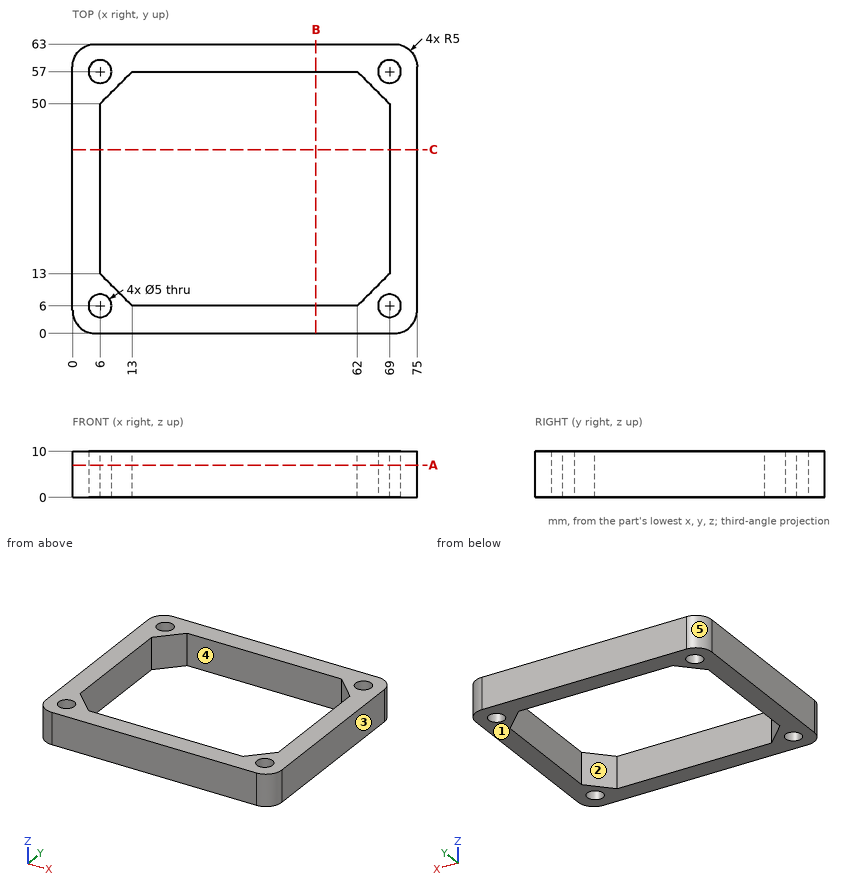
Can you work these out from the drawing? Everything is in mm from the part's minimum corner. A direction names the side the tool comes from. Give positions to 0.01 mm unless a question says otherwise; leave off trailing zeros. Order: outer loops, then holes, each group sorted by start corner. A loop starts at its lowest first (then second) coordinate and runs counter-clockwise, first axis right, second up. Notation, with made-up numbers: M 66.5,24.5 L 99.5,24.5 A22 ccw 99.5,60.5 Z; hole C 53.5,0 d10. An arc over 180 degrees is marked long. Use a Markdown table: item, result. Add a question column.
1. Suppose I cut it at A-A (z = 7). List the corners of the cut face in (x, y) for me, and give its area (3 significant figures).
2. Suppose I cut it at C-C (y = 40). List the corners of the cut face in (x, z) for me.
3. I need wall thicknesses on probe 1 along X at (y, z) = (46, 2.75); probe 2 along Y at (x, z) = (32.5, 8); probe 3 along X at (y, z) = (59, 7.25). Which ranges of each line are inside material? Lowest first, please. Write a range as from..to.
4. If we mould it in two halves opening along Y, with no side actions, what happens to the marked faces 3, 4 and 5? For each: +Y half, -Y half, draft (parallel to the pull), parting line (faces both ways), or undercut.
5. On a 3-axis mill with a long thin cutter (end or side, diameter ignored), from which of +Z, -Z, +X, -X, +Y, -Y can I reach the whole of each face in a straight line? I mean the marked faces 1 and 2. Say none if no direction works.
6. For pin 1 Ø3 at (x, y) = (69, 57) entering from -Z, with a flat end and sliding along its axis, tell me the tip position at first contact or that it passes through.
7. Suppose I cut it at B-B (x = 53). List the corners of the cut face in (y, z) for me, and give its area (3 significant figures).
Results list:
| question | item | result |
|---|---|---|
| 1 | outline | M 0,5 A5 ccw 5,0 L 70,0 A5 ccw 75,5 L 75,58 A5 ccw 70,63 L 5,63 A5 ccw 0,58 Z; hole C 6,6 d5; hole C 6,57 d5; hole M 6,13 L 13,6 L 62,6 L 69,13 L 69,50 L 62,57 L 13,57 L 6,50 Z; hole C 69,6 d5; hole C 69,57 d5 |
| 1 | area | 1,510 mm² |
| 2 | outline | M 0,0 L 6,0 L 6,10 L 0,10 Z; M 69,0 L 75,0 L 75,10 L 69,10 Z |
| 3 | probe 1 | x = 0..6, 69..75 |
| 3 | probe 2 | y = 0..6, 57..63 |
| 3 | probe 3 | x = 0.1..4.5, 7.5..67.5, 70.5..74.9 |
| 4 | face 3 | draft |
| 4 | face 4 | undercut |
| 4 | face 5 | +Y half |
| 5 | face 1 | -Z, +X, -X, +Y, -Y |
| 5 | face 2 | +Z, -Z |
| 6 | pin 1 | passes through |
| 7 | outline | M 0,0 L 6,0 L 6,10 L 0,10 Z; M 57,0 L 63,0 L 63,10 L 57,10 Z |
| 7 | area | 120 mm² |
